Here's how the part is built. I have some questions about the finished solid (model axes, mm). A direction names the side the tool comes from. Round coordinates to 2 decimals unless told otherwise and drop trailing zeros. Write each loop counter-clockwise with the first axis right and the second up, starting at its lowest first coordinate (ties: lowest second). Pieces come first, ordered by that corner, then holes. Notation, with made-up numbers: M 79.25,66.25 L 132.25,66.25 A32 ccw 132.25,97.25 Z; hole C 80,20.5 d3. An arc over 180 degrees is marked long. Use a Markdown table: item, result. Add a question column.
```python
from build123d import *

# Parameters (mm, degrees)
SKETCH1_W            = 225.25
SKETCH1_H            = 12.5
BOSS_EXTRUDE1_DEPTH  = 133.58
CUT_EXTRUDE1_DEPTH   = 159.09
SKETCH11_W           = 88.5
SKETCH11_H           = 154.09
CUT_EXTRUDE2_DEPTH   = 176.169223966
SKETCH12_W           = 13
SKETCH12_H           = 17.045
CUT_EXTRUDE3_DEPTH   = 2
M4_CLEARANCE_HOLE1_D = 4.5
BOSS_EXTRUDE3_DEPTH  = 154.09
CHAMFER4_START       = -19.51
CHAMFER4_DEPTH       = 154.51
CHAMFER5_START       = -19.51
CHAMFER5_DEPTH       = 154.51
CUT_EXTRUDE4_DEPTH   = 1.75
BOSS_EXTRUDE4_DEPTH  = 1.5
CUT_EXTRUDE5_DEPTH   = 176.169223966
CHAMFER6_SIZE        = 5
SKETCH19_W           = 155
SKETCH19_H           = 10
BOSS_EXTRUDE5_DEPTH  = 15
M4_CLEARANCE_HOLE2_D = 4.5


with BuildPart() as part:
    # Sketch1 → Boss-Extrude1 (new, symmetric)
    with BuildSketch(Plane.XY):
        with Locations((0, 6.25)):
            Rectangle(SKETCH1_W, SKETCH1_H)
    extrude(amount=BOSS_EXTRUDE1_DEPTH, both=True)

    # Sketch4 → Cut-Extrude1 (cut)
    with BuildSketch(Plane.XY.offset(133.58)):
        Polygon((-59.125, 12.5), (-59.125, 9.5), (-62.125, 9.5), (-62.125, 5), (-40.125, 5), (-40.125, 9.5), (-43.125, 9.5), (-43.125, 12.5), align=None)
        Polygon((63.375, 12.5), (63.375, 9.5), (60.375, 9.5), (60.375, 5), (82.375, 5), (82.375, 9.5), (79.375, 9.5), (79.375, 12.5), align=None)
    extrude(amount=-CUT_EXTRUDE1_DEPTH, mode=Mode.SUBTRACT)

    # Sketch11 → Cut-Extrude2 (cut, through all)
    with BuildSketch(Plane(origin=(0, 12.5, 0), x_dir=(1, 0, 0), z_dir=(0, 1, 0))):
        with Locations((10.125, -56.535)):
            Rectangle(SKETCH11_W, SKETCH11_H)
    extrude(amount=-CUT_EXTRUDE2_DEPTH, mode=Mode.SUBTRACT)

    # Sketch12 → Cut-Extrude3 (cut)
    with BuildSketch(Plane(origin=(0, 12.5, 0), x_dir=(1, 0, 0), z_dir=(0, 1, 0))):
        with Locations((-83.375, -125.0575)):
            Rectangle(SKETCH12_W, SKETCH12_H)
        with Locations((95, -125.0575)):
            Rectangle(SKETCH12_W, SKETCH12_H)
    extrude(amount=-CUT_EXTRUDE3_DEPTH, mode=Mode.SUBTRACT)

    # M4 Clearance Hole1 (through all)
    with Locations(Plane(origin=(0, 10.5, 0), x_dir=(1, 0, 0), z_dir=(0, 1, 0))):
        with Locations((-83.375, -126.535), (95, -126.535)):
            Hole(M4_CLEARANCE_HOLE1_D / 2)

    # Sketch15 → Boss-Extrude3 (add)
    with BuildSketch(Plane.XY.offset(133.58)):
        Polygon((-34.125, 0), (-21.625, 0), (-21.625, 8), (-26.625, 8), (-34.125, 12.5), align=None)
        Polygon((54.375, 0), (41.875, 0), (41.875, 8), (46.875, 8), (54.375, 12.5), align=None)
    extrude(amount=-BOSS_EXTRUDE3_DEPTH)

    # Chamfer4: read off the stored shape, not the designer's step
    # Chamfer4 outline → Chamfer4 (cut)
    with BuildSketch(Plane.XY.offset(CHAMFER4_START)):
        Polygon((-112.625, 12.5), (-112.625, 7.5), (-107.625, 12.5), align=None)
    extrude(amount=CHAMFER4_DEPTH, mode=Mode.SUBTRACT)

    # Chamfer5: read off the stored shape, not the designer's step
    # Chamfer5 outline → Chamfer5 (cut)
    with BuildSketch(Plane.XY.offset(CHAMFER5_START)):
        Polygon((112.625, 12.5), (107.625, 12.5), (112.625, 7.5), align=None)
    extrude(amount=CHAMFER5_DEPTH, mode=Mode.SUBTRACT)

    # Sketch16 → Cut-Extrude4 (cut, symmetric)
    with BuildSketch(Plane(origin=(0, 4.25, 0), x_dir=(-1, 0, 0), z_dir=(0, -1, 0))):
        with BuildLine():
            Line((21.625, -126.452281323), (21.625, -120.707718677))
            ThreePointArc((21.625, -120.707718677), (23.125, -123.58), (21.625, -126.452281323))
        make_face()
        with BuildLine():
            Line((-41.875, -120.707718677), (-41.875, -126.452281323))
            ThreePointArc((-41.875, -126.452281323), (-43.375, -123.58), (-41.875, -120.707718677))
        make_face()
    extrude(amount=CUT_EXTRUDE4_DEPTH, both=True, mode=Mode.SUBTRACT)

    # Sketch17 → Boss-Extrude4 (add, symmetric)
    with BuildSketch(Plane(origin=(0, 4.25, 0), x_dir=(-1, 0, 0), z_dir=(0, -1, 0))):
        with BuildLine():
            Line((-41.875, 3.382281323), (-41.875, -2.362281323))
            ThreePointArc((-41.875, -2.362281323), (-40.375, 0.51), (-41.875, 3.382281323))
        make_face()
        with BuildLine():
            Line((21.625, -2.362281323), (21.625, 3.382281323))
            ThreePointArc((21.625, 3.382281323), (20.125, 0.51), (21.625, -2.362281323))
        make_face()
    extrude(amount=BOSS_EXTRUDE4_DEPTH, both=True)

    # Sketch18 → Cut-Extrude5 (cut, through all)
    with BuildSketch(Plane(origin=(0, 12.5, 0), x_dir=(1, 0, 0), z_dir=(0, 1, 0))):
        Polygon((87.625, 45.51), (-67.375, 45.51), (-67.375, 25.51), (-112.625, 25.51), (-112.625, 133.58), (112.625, 133.58), (112.625, 25.51), (87.625, 25.51), align=None)
    extrude(amount=-CUT_EXTRUDE5_DEPTH, mode=Mode.SUBTRACT)

    # Chamfer6
    # the kernel refuses this chamfer: 5 mm, written as the material it takes off along each edge
    with BuildSketch(Plane(origin=(67.23341494, 12.5, -20.51), x_dir=(0, -1, 0), z_dir=(-1, 0, 0))) as chamfer6_piece_1_section:
        Polygon((CHAMFER6_SIZE, 0), (0, -CHAMFER6_SIZE), (0, 0), align=None)
    chamfer6_piece_1 = extrude(amount=114.21682988, mode=Mode.PRIVATE)
    chamfer6_piece_1 = split(chamfer6_piece_1, bisect_by=Plane(origin=(41.875, 12.5, -20.51), z_dir=(1, 0, 0)), keep=Keep.TOP, mode=Mode.PRIVATE)
    chamfer6_piece_1 = split(chamfer6_piece_1, bisect_by=Plane(origin=(67.23341494, 8, -20.51), z_dir=(0, 1, 0)), keep=Keep.TOP, mode=Mode.PRIVATE)
    chamfer6_piece_1 = split(chamfer6_piece_1, bisect_by=Plane(origin=(63.829716868, 18.172830121, -20.51), z_dir=(-0.514495755427524, 0.8574929257125457, 0)), keep=Keep.TOP, mode=Mode.PRIVATE)
    add(chamfer6_piece_1, mode=Mode.SUBTRACT)
    with BuildSketch(Plane(origin=(67.23341494, 12.5, -20.51), x_dir=(0, -1, 0), z_dir=(-1, 0, 0))) as chamfer6_piece_2_section:
        Polygon((CHAMFER6_SIZE, 0), (0, -CHAMFER6_SIZE), (0, 0), align=None)
    chamfer6_piece_2 = extrude(amount=114.21682988, mode=Mode.PRIVATE)
    chamfer6_piece_2 = split(chamfer6_piece_2, bisect_by=Plane(origin=(41.875, 12.5, -20.51), z_dir=(-1, 0, 0)), keep=Keep.TOP, mode=Mode.PRIVATE)
    chamfer6_piece_2 = split(chamfer6_piece_2, bisect_by=Plane(origin=(67.23341494, 8, -20.51), z_dir=(0, -1, 0)), keep=Keep.TOP, mode=Mode.PRIVATE)
    chamfer6_piece_2 = split(chamfer6_piece_2, bisect_by=Plane(origin=(-21.625, 12.5, -20.51), z_dir=(1, 0, 0)), keep=Keep.TOP, mode=Mode.PRIVATE)
    add(chamfer6_piece_2, mode=Mode.SUBTRACT)
    with BuildSketch(Plane(origin=(67.23341494, 12.5, -20.51), x_dir=(0, -1, 0), z_dir=(-1, 0, 0))) as chamfer6_piece_3_section:
        Polygon((CHAMFER6_SIZE, 0), (0, -CHAMFER6_SIZE), (0, 0), align=None)
    chamfer6_piece_3 = extrude(amount=114.21682988, mode=Mode.PRIVATE)
    chamfer6_piece_3 = split(chamfer6_piece_3, bisect_by=Plane(origin=(41.875, 12.5, -20.51), z_dir=(-1, 0, 0)), keep=Keep.TOP, mode=Mode.PRIVATE)
    chamfer6_piece_3 = split(chamfer6_piece_3, bisect_by=Plane(origin=(67.23341494, 8, -20.51), z_dir=(0, 1, 0)), keep=Keep.TOP, mode=Mode.PRIVATE)
    chamfer6_piece_3 = split(chamfer6_piece_3, bisect_by=Plane(origin=(-21.625, 12.5, -20.51), z_dir=(1, 0, 0)), keep=Keep.TOP, mode=Mode.PRIVATE)
    add(chamfer6_piece_3, mode=Mode.SUBTRACT)
    with BuildSketch(Plane(origin=(67.23341494, 12.5, -20.51), x_dir=(0, -1, 0), z_dir=(-1, 0, 0))) as chamfer6_piece_4_section:
        Polygon((CHAMFER6_SIZE, 0), (0, -CHAMFER6_SIZE), (0, 0), align=None)
    chamfer6_piece_4 = extrude(amount=114.21682988, mode=Mode.PRIVATE)
    chamfer6_piece_4 = split(chamfer6_piece_4, bisect_by=Plane(origin=(40.403246279, -32.216947768, -20.51), z_dir=(0.5144957554275245, 0.8574929257125454, 0)), keep=Keep.TOP, mode=Mode.PRIVATE)
    chamfer6_piece_4 = split(chamfer6_piece_4, bisect_by=Plane(origin=(67.23341494, 8, -20.51), z_dir=(0, 1, 0)), keep=Keep.TOP, mode=Mode.PRIVATE)
    chamfer6_piece_4 = split(chamfer6_piece_4, bisect_by=Plane(origin=(-21.625, 12.5, -20.51), z_dir=(-1, 0, 0)), keep=Keep.TOP, mode=Mode.PRIVATE)
    add(chamfer6_piece_4, mode=Mode.SUBTRACT)

    # Sketch19 → Boss-Extrude5 (add)
    with BuildSketch(Plane(origin=(0, 12.5, 0), x_dir=(1, 0, 0), z_dir=(0, 1, 0))):
        with Locations((10.125, 40.51)):
            Rectangle(SKETCH19_W, SKETCH19_H)
    extrude(amount=BOSS_EXTRUDE5_DEPTH)

    # M4 Clearance Hole2 (through all)
    with Locations(Plane.XY.offset(-35.51)):
        with Locations((-19.875, 18.75), (40.125, 18.75)):
            Hole(M4_CLEARANCE_HOLE2_D / 2)


solid = part.part
```
Item 1: Imagine slicing it at B-B on x = 10. List the corners of the cut face in (y, z) for me.
Item 2: If we mould it in two halves opening along Y, with no side actions, what happens to faces 1 (the face through (-40.125, 7, 55)), 2 (the face through (-83, 10.5, 123)), 3 (the face through (-85.45, 5.18, 127.4))? For each: +Y half, -Y half, draft (parallel to the pull), parting line (faces both ways), or undercut.
Item 3: I need wall thicknesses on probe 1 along X at (y, z) = (6.25, -2) (3 decimals); probe 2 along Y at (x, z) = (-22, 83.5); probe 3 along Y at (x, z) = (-53, -3.5). Which ranges of each line are inside material? Lowest first, please. Write a range as from..to.
Item 4: For pin 1 Ø3.5 at (x, y) = (40.125, 18.75) entering from +Z; pin 2 Ø6 at (x, z) = (-65.5, 15.5) entering from -Y; pin 3 Ø0.8 at (x, z) = (-21, -0.5) entering from +Y; pin 4 Ø1.5 at (y, z) = (11.5, 29.5) entering from -X (3 decimals), each with a flat end and sliding along its axis, tell me the tip position at first contact or that it passes through.
Item 5: On a 3-axis mill with a long thin cutter (end or side, diameter ignored), from which of +Z, -Z, +X, -X, +Y, -Y can I reach the whole of each face in a straight line? I mean faces 4 (the face through (110.09, 10.035, 55.963)), 5 (the face through (44, 8, 57)), 6 (the face through (-42, 12.5, 43)), 7 (the face through (-51, 5, 55)), 8 (the face through (-67.375, 11, -38)). Say none if no direction works.
Item 6: Imagine slicing it at C-C on z = -29. List the corners of the cut face in (x, y) for me (3 decimals), plus the area to 3 significant figures.
Item 7: Imagine slicing it at D-D on x = -97. List the corners of the cut face in (y, z) for me, plus the area to 3 significant figures.
The answers:
| question | item | result |
|---|---|---|
| 1 | outline | M 0,-45.51 L 27.5,-45.51 L 27.5,-35.51 L 12.5,-35.51 L 12.5,-25.51 L 7.5,-20.51 L 0,-20.51 Z |
| 2 | face 1 | undercut |
| 2 | face 2 | +Y half |
| 2 | face 3 | draft |
| 3 | probe 1 | -112.625..-62.125, -40.125..-21.625, 41.875..60.375, 82.375..112.625 |
| 3 | probe 2 | 0..8 |
| 3 | probe 3 | 0..5 |
| 4 | pin 1 | through |
| 4 | pin 2 | y = 0 |
| 4 | pin 3 | y = 5.75 |
| 4 | pin 4 | x = -109.375 |
| 5 | face 4 | +Z, +X, +Y |
| 5 | face 5 | +Z, +Y |
| 5 | face 6 | +Z, +X, -X, +Y |
| 5 | face 7 | +Z |
| 5 | face 8 | -Z, -X, +Y, -Y |
| 6 | outline | M -67.375,0 L 87.625,0 L 87.625,12.5 L -67.375,12.5 Z |
| 6 | area | 1,940 mm² |
| 7 | outline | M 0,-25.51 L 12.5,-25.51 L 12.5,133.58 L 0,133.58 Z |
| 7 | area | 1,990 mm² |
